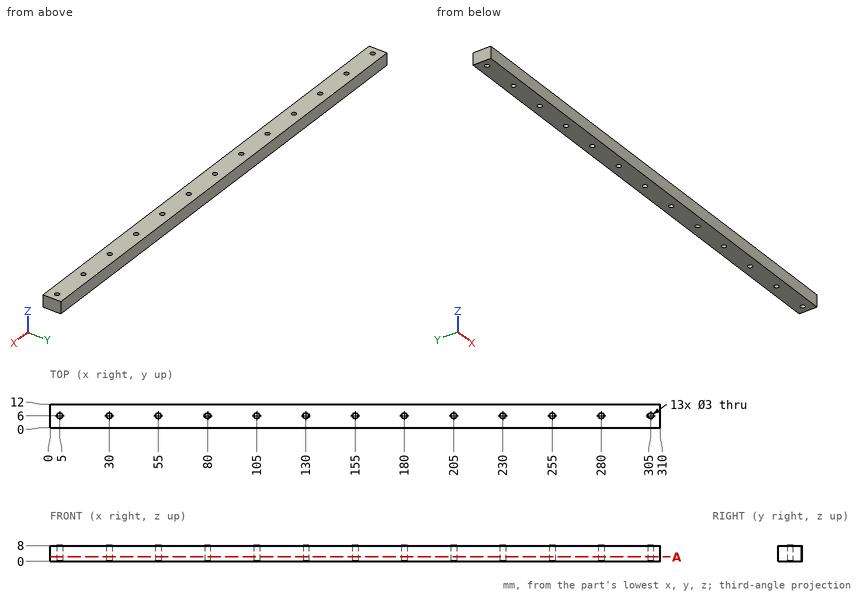
Answer from the drawing. Dimensions are ordinates in mm from the lowest x, y and z of the part. Coordinates: 2 decimals unless noted, no trailing zeros. Answer as a JSON object with one key per item and string values. Group by question number.
Item 1: Section A-A (z = 2.25) is taken. State how many separate pieces and enclosed holes the cut face has, plus the area to 3 significant figures.
Item 2: Consider probe 1 along Y at (x, z) = (80, 5.75); probe 2 along Y at (x, z) = (279.5, 4.75). Determine where each line is inside the solid, lowest interval first. Write a range as from..to.
Item 3: A flat-ended cylindrical pin translates along its axis: P1, Ø5, axis at x = 180, y = 6, coming from the +Z side. Find the tip coordinate at first contact, or state that the pin passes through.
Results are:
{
 "1": {"separate pieces": "1", "enclosed holes": "13", "area": "3,630 mm^2"},
 "2": {"probe 1": "y = 0..4.5, 7.5..12", "probe 2": "y = 0..4.59, 7.41..12"},
 "3": {"P1": "stops at z = 8"}
}
